Autodesk Inventor part; units mm, degrees
ref_plane "YZ Plane" through (0, 0, 0) normal (1, 0, 0) x (0, 1, 0)
ref_plane "XZ Plane" through (0, 0, 0) normal (0, 1, 0) x (-1, 0, 0)
ref_plane "XY Plane" through (0, 0, 0) normal (0, 0, 1) x (1, 0, 0)
sketch "Skizze1" plane through (0, 0, 0) normal (0, 1, 0) x (-1, 0, 0)
  line L0 (35.5112, -88.3128) -> (35.5112, -108.3128)
  line L1 (35.5112, -108.3128) -> (22.0645, -123.1178)
  line L2 (22.0645, -123.1178) -> (2.0645, -123.1178)
  line L3 (2.0645, -123.1178) -> (-12.7404, -109.6711)
  line L4 (-12.7404, -109.6711) -> (-12.7404, -89.6711)
  line L5 (-12.7404, -89.6711) -> (0.7063, -74.8661)
  line L6 (0.7063, -74.8661) -> (20.7063, -74.8661)
  line L7 (20.7063, -74.8661) -> (35.5112, -88.3128)
  point P0 (0, 0)
  dimension "d0" = 20
  dimension "d1" = 20
  dimension "d2" = 20
  dimension "d3" = 20
  dimension "d4" = 20
  dimension "d5" = 20
  dimension "d6" = 20
  dimension "d7" = 20
extrude "Extrusion1" add sketch "Skizze1" along normal blind 5
sketch "Skizze2" plane through (-2.0645, 0, -123.1178) normal (0, 0, -1) x (-1, 0, 0)
  circle A0 centre (10, 2.5) radius 2.5
  line L0 (0, 5) -> (20, 5)
  point P0 (-2.0645, 0)
  dimension "d11" = 5
  dimension "d12" = 2.5
extrude "Extrusion2" add sketch "Skizze2" along normal blind 81.748
sketch "Skizze3" plane through (-12.0645, 2.5, -204.8658) normal (0, 0, -1) x (-1, 0, 0)
  line L0 (-35, -15) -> (35, -15)
  line L1 (35, -15) -> (35, 15)
  line L2 (35, 15) -> (-35, 15)
  line L3 (-35, 15) -> (-35, -15)
  arc A0 (0, -2.5) -> (0, 2.5) centre (0, 0) ccw
  line L4 (-35, -15) -> (35, 15) construction
  line L5 (35, -15) -> (-35, 15) construction
  point P0 (-12.0645, -2.5)
  point P1 (-2.7951, -2.5)
  point P2 (-2.7951, 2.5)
  dimension "d15" = 70
  dimension "d16" = 30
extrude "Extrusion3" add sketch "Skizze3" against normal blind 2
properties part number "Stoppschild"
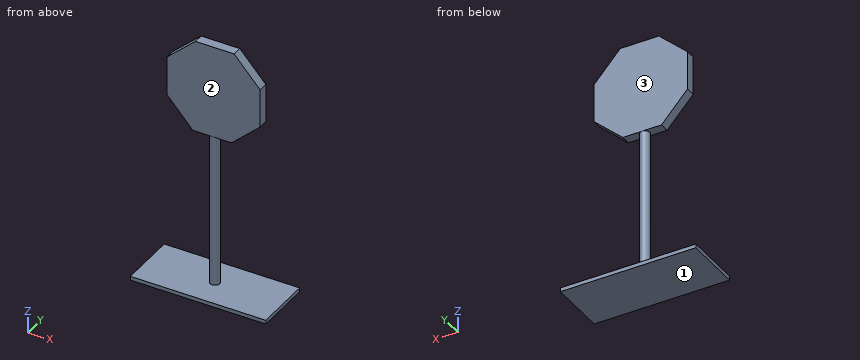
Geometry: final body of the model. Coordinates: model frame, mm. Face numbers are marked on the shaded views. A direction names the side the tool comes from. Give positions to 0.01 mm unless a question says otherwise; leave off trailing zeros. Write each loop counter-clockwise with the first axis right and the second up, starting at its lowest first coordinate (ties: lowest second). Pieces come first, ordered by that corner, then holes.
1. Line query: probe 1 along Z at (x, y) = (-5, -1.75); probe 2 along Z at (x, y) = (-20.5, 4.5); probe 3 along Y at (x, z) = (-14, -101). Output: solid intervals per line, ascending.
2. Reachability of the marked faces 1, 2 and 3 from +Z, -Z, +X, -X, +Y, -Y: full face, straight path, thin tool, end or side. Return the list, or none.
3. Pin query (flat end, axial travel): P1, Ø14.5, axis at x = -11, z = -103, coming from the +Y side; P2, Ø2, axis at x = -11, y = -8.5, coming from the +Z side; P3, Ø1.5, axis at y = 3, z = -95, coming from the +X side. Return the tip coordinate at first contact, or that it passes through.
4. Section query B-B, the plane y = 2.5. Return loops of the section in (x, z), then the cut area to 3 significant figures.
5. Section query D-D, the plane z = -105. Return loops of the section in (x, y), then the cut area to 3 significant figures.
6. Section query A-A, the plane x = 8.5. Return loops of the section in (y, z).
7. Section query C-C, the plane z = -187. Return loops of the section in (x, y), then the cut area to 3 significant figures.
Computed:
1. probe 1: z = -204.87 to -202.87
1. probe 2: z = -204.87 to -202.87, -123.12 to -74.87
1. probe 3: y = 0 to 5
2. face 1: -Z, +X, -X, +Y, -Y
2. face 2: +Z, +X, -X, -Y
2. face 3: +Z, +X, -X, +Y
3. P1: stops at y = 5
3. P2: stops at z = -202.87
3. P3: stops at x = 12.74
4. outline: (-47.06, -204.87) - (22.94, -204.87) - (22.94, -202.87) - (-9.56, -202.87) - (-9.56, -123.12) - (-2.06, -123.12) - (12.74, -109.67) - (12.74, -89.67) - (-0.71, -74.87) - (-20.71, -74.87) - (-35.51, -88.31) - (-35.51, -108.31) - (-22.06, -123.12) - (-14.56, -123.12) - (-14.56, -202.87) - (-47.06, -202.87) - close
4. area: 2,470 mm2
5. outline: (-35.51, 0) - (12.74, 0) - (12.74, 5) - (-35.51, 5) - close
5. area: 241 mm2
6. outline: (-12.5, -204.87) - (17.5, -204.87) - (17.5, -202.87) - (-12.5, -202.87) - close; (0, -113.52) - (5, -113.52) - (5, -85) - (0, -85) - close
7. outline: circle Ø5 at (-12.06, 2.5)
7. area: 19.6 mm2
